Design review of the part built by this model. Coordinates are the model's own, in mm. A direction names the side the tool comes from. Round coordinates to 2 decimals unless told otherwise and drop trailing zeros. Write each loop counter-clockwise with the first axis right and the second up, starting at its lowest first coordinate (ties: lowest second). Pieces come first, ordered by that corner, then holes.
from build123d import *

# Parameters (mm, degrees)
SKETCH_W     = 120.3
SKETCH_H     = 40.2
SKETCH_R     = 1.5
SKETCH_R_2   = 3
PAD_DEPTH    = 3
POCKET_DEPTH = 1.5


with BuildPart() as part:
    # Sketch → Pad (new body)
    with BuildSketch(Plane.XY):
        Rectangle(SKETCH_W, SKETCH_H)
        with Locations((-12.5, 9.6)):
            Circle(SKETCH_R, mode=Mode.SUBTRACT)
        with Locations((12.5, 9.6)):
            Circle(SKETCH_R, mode=Mode.SUBTRACT)
        with Locations((43.15, -12.1)):
            Circle(SKETCH_R_2, mode=Mode.SUBTRACT)
        with Locations((33.15, -12.1)):
            Circle(SKETCH_R_2, mode=Mode.SUBTRACT)
        with Locations((23.15, -12.1)):
            Circle(SKETCH_R_2, mode=Mode.SUBTRACT)
        with Locations((13.15, -12.1)):
            Circle(SKETCH_R_2, mode=Mode.SUBTRACT)
        with Locations((3.15, -12.1)):
            Circle(SKETCH_R_2, mode=Mode.SUBTRACT)
        with Locations((-6.85, -12.1)):
            Circle(SKETCH_R_2, mode=Mode.SUBTRACT)
        with Locations((-33.15, -12.1)):
            Circle(SKETCH_R_2, mode=Mode.SUBTRACT)
        with Locations((-43.15, -12.1)):
            Circle(SKETCH_R_2, mode=Mode.SUBTRACT)
        with BuildLine():
            Line((28.4, 1.325), (34.9, 1.325))
            ThreePointArc((34.9, 1.325), (35.196827, 1.42264), (35.377726, 1.677426))
            Line((35.377726, 1.677426), (36.15, 4.177426))
            ThreePointArc((36.15, 4.177426), (36.074634, 4.621827), (35.672274, 4.825))
            Line((35.672274, 4.825), (27.627726, 4.825))
            ThreePointArc((27.627726, 4.825), (27.225366, 4.621827), (27.15, 4.177426))
            Line((27.15, 4.177426), (27.922274, 1.677426))
            ThreePointArc((27.922274, 1.677426), (28.103173, 1.42264), (28.4, 1.325))
        make_face(mode=Mode.SUBTRACT)
        with BuildLine():
            Line((-7.25, 14.6), (7.25, 14.6))
            ThreePointArc((9.672278, 11.481477), (9.224374, 13.633573), (7.25, 14.6))
            Line((8.203367, 5.728886), (9.672278, 11.481477))
            ThreePointArc((6.75, 4.6), (7.670144, 4.915375), (8.203367, 5.728886))
            Line((6.75, 4.6), (-6.75, 4.6))
            ThreePointArc((-8.203367, 5.728886), (-7.670144, 4.915375), (-6.75, 4.6))
            Line((-8.203367, 5.728886), (-9.672278, 11.481477))
            ThreePointArc((-7.25, 14.6), (-9.224374, 13.633573), (-9.672278, 11.481477))
        make_face(mode=Mode.SUBTRACT)
    extrude(amount=PAD_DEPTH)

    # Sketch001 (on Face32 of Pad) → Pocket (cut)
    with BuildSketch(Plane.XY.offset(3)):
        with BuildLine():
            ThreePointArc((27.7, 7.13), (23.7, 3.13), (27.7, -0.87))
            Line((27.7, -0.87), (35.7, -0.87))
            ThreePointArc((35.7, -0.87), (39.7, 3.13), (35.7, 7.13))
            Line((35.7, 7.13), (27.7, 7.13))
        make_face()
    extrude(amount=-POCKET_DEPTH, mode=Mode.SUBTRACT)


solid = part.part
1) For line 1 along X through (y, z) = (3, 2.45); line 2 along Y through (x, z) = (2, 1.5); line 3 along Y through (x, z) = (25.5, 2.65), list the stretches that pass through material, from the lowest coordinate up.
2) Add section C-C on x = 2. State the section outline as (y, z) points.
3) The part is to be moulded in two halves that separate along Y. For faces 4 (the face through (-1, 20.1, 1)), 5 (the face through (34.534, -14.762, 1.479)), 6 (the face through (-1, 0, 3)), say which applies: pulls with the +Y half, pulls with the -Y half, needs draft (parallel to the pull), parting line crosses it, or undercut.
4) For faces 1 (the face through (60.15, 0, 1)), 2 (the face through (0, 14.6, 1)), 3 (the face through (23.7, 3.2, 2.3)), list the 3-axis set-ups (+Z, -Z, +X, -X, +Y, -Y) from which the entire face can be reached by the end or side of a thin tool; tool diameter is ignored.
5) Add section A-A on x = -43.15. State the section outline as (y, z) points.
6) Add section B-B on z = 2.45. Count the separate pieces of the cut face and the enclosed holes in it, and give its area (3 significant figures).
Computed:
1. line 1: x = -60.15 to 23.7, 39.7 to 60.15
1. line 2: y = -20.1 to -14.87, -9.33 to 4.6, 14.6 to 20.1
1. line 3: y = -20.1 to -13.96, -10.24 to -0.21, 6.47 to 20.1
2. outline: (-20.1, 0) - (-14.87, 0) - (-14.87, 3) - (-20.1, 3) - close; (-9.33, 0) - (4.6, 0) - (4.6, 3) - (-9.33, 3) - close; (14.6, 0) - (20.1, 0) - (20.1, 3) - (14.6, 3) - close
3. face 4: pulls with the +Y half
3. face 5: undercut
3. face 6: needs draft
4. face 1: +Z, -Z, +X, +Y, -Y
4. face 2: +Z, -Z
4. face 3: +Z
5. outline: (-20.1, 0) - (-15.1, 0) - (-15.1, 3) - (-20.1, 3) - close; (-9.1, 0) - (20.1, 0) - (20.1, 3) - (-9.1, 3) - close
6. separate pieces: 1
6. enclosed holes: 12
6. area: 4,300 mm2
